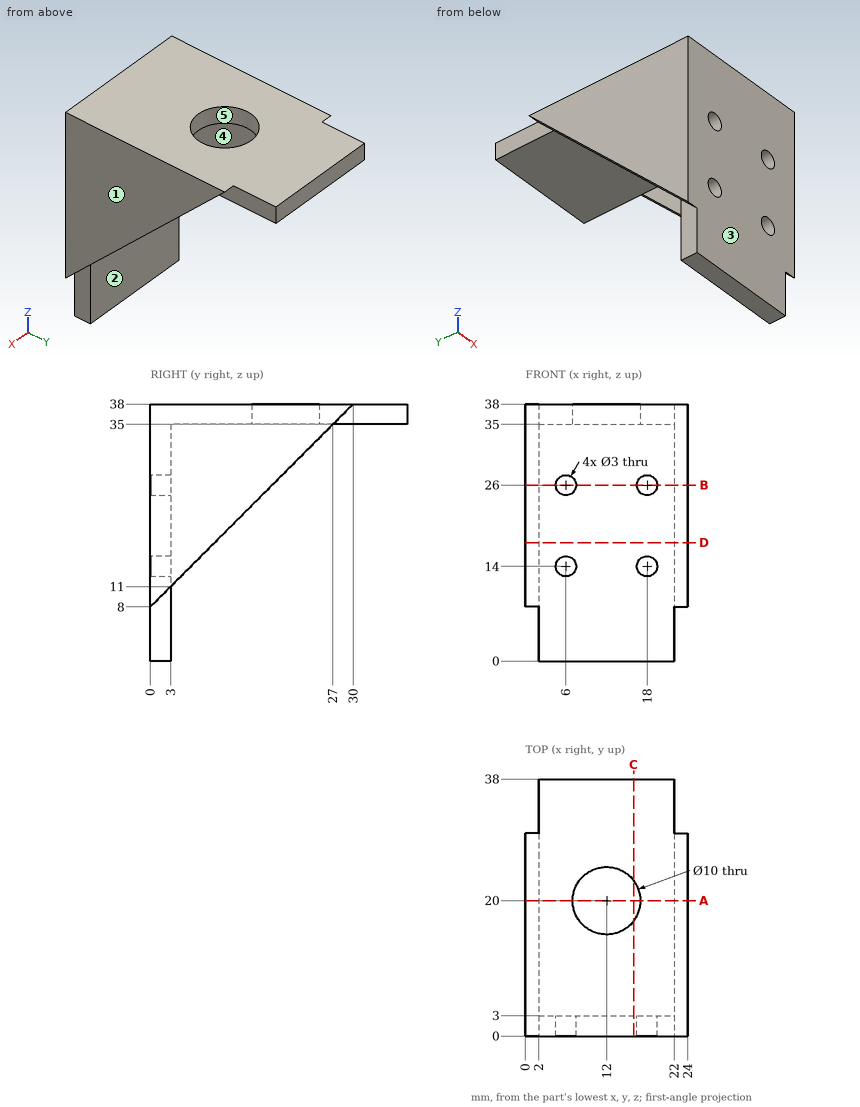
The figure shows three views and two pictorial views of one solid part (mm, origin at its lowest corner). Answer the questions. A direction names the side the tool comes from. Round coordinates to 2 decimals unless told otherwise and drop trailing zeros. Write each loop counter-clockwise with the first axis right and the second up, starting at its lowest first coordinate (ties: lowest second). Pieces come first, ordered by that corner, then holes. Notation, with made-up numbers: M 18.5,37.25 L 63.5,37.25 A19 cw 63.5,70.25 Z; hole C -9.5,-3 d7. An arc over 180 degrees is marked long. Use a Markdown table: item, result.
1) For a pull along X with two mould halves and no side action, classify the marked faces 1, 2 and 3 as pulls with the +X half, pulls with the -X half, needs draft (parallel to the pull), parting line crosses it, or undercut.
Answers follow:
| item | result |
|---|---|
| face 1 | pulls with the +X half |
| face 2 | undercut |
| face 3 | needs draft |
2) The part is cut by section D-D (z = 17.5). Write down the section's boundary in (x, y).
Answers follow:
| item | result |
|---|---|
| outline | M 0,0 L 24,0 L 24,9.5 L 22,9.5 L 22,3 L 2,3 L 2,9.5 L 0,9.5 Z |
3) The part is cut by section C-C (x = 16). Write down the section's boundary in (y, z).
Answers follow:
| item | result |
|---|---|
| outline | M 0,0 L 3,0 L 3,35 L 17,35 L 17,38 L 0,38 Z; M 23,35 L 38,35 L 38,38 L 23,38 Z |
4) Flat-ended cylindrical pins translate along their axes: pin 1 (0.9 mm diameter, centred on y = 33.5, z = 36.5, fed in from +X); pin 2 (1.5 mm diameter, centred on y = 34, z = 37, fed in from -X); pin 3 (6 mm diameter, centred on x = 15.5, y = 20, fed in from -Z). Find the tip coordinate at first contact, or state that the pin passes through.
Answers follow:
| item | result |
|---|---|
| pin 1 | stops at x = 22 |
| pin 2 | stops at x = 2 |
| pin 3 | stops at z = 35 |
5) The part is cut by section A-A (y = 20). Write down the section's boundary in (x, z).
Answers follow:
| item | result |
|---|---|
| outline | M 0,28 L 2,28 L 2,35 L 7,35 L 7,38 L 0,38 Z; M 17,35 L 22,35 L 22,28 L 24,28 L 24,38 L 17,38 Z |
6) A tool of negligible diameter and unlimited length cuts with its end or side. For the marked faces 4 and 5, from which of +Z, -Z, +X, -X, +Y, -Y can it reach the whole face along a straight path? Write none if from no direction.
Answers follow:
| item | result |
|---|---|
| face 4 | -Z, +Y |
| face 5 | +Z, -Z |
7) Straight lines are drawn through the part: line 1 along X through (y, z) = (1.25, 26); line 2 along X through (y, z) = (7, 33); line 3 along Y through (x, z) = (12, 35.6). For each, find the intervals that lie inside material, in ascending order. Write a range as [from, to].
Answers follow:
| item | result |
|---|---|
| line 1 | x = [0, 4.5], [7.5, 16.5], [19.5, 24] |
| line 2 | x = [0, 2], [22, 24] |
| line 3 | y = [0, 15], [25, 38] |
8) The part is cut by section B-B (z = 26). Write down the section's boundary in (x, y), plus the area to 3 significant figures.
Answers follow:
| item | result |
|---|---|
| outline | M 0,0 L 4.5,0 L 4.5,3 L 2,3 L 2,18 L 0,18 Z; M 7.5,0 L 16.5,0 L 16.5,3 L 7.5,3 Z; M 19.5,0 L 24,0 L 24,18 L 22,18 L 22,3 L 19.5,3 Z |
| area | 114 mm2 |
